Design review of the part built by this model. Coordinates are the model's own, in mm. A direction names the side the tool comes from. Round coordinates to 2 decimals unless told otherwise and drop trailing zeros. Order: outer loops, then holes, each group sorted by start corner. A loop starts at its lowest first (then second) coordinate and runs counter-clockwise, first axis right, second up. Notation, with made-up numbers: (83.25, -32) - (140.25, -32) arc R7 cw to (140.25, -22) - close; hole circle Ø6 at (62.5, 15). An arc over 180 degrees is marked (long way). Write item = value, one per line.
from build123d import *

# Parameters (mm, degrees)
SKETCH4_R           = 1.016
BOSS_EXTRUDE3_DEPTH = 8.382
BOSS_EXTRUDE4_DEPTH = 12.7
FILLET4_R           = 9.652


with BuildPart() as part:
    # Sketch4 → Boss-Extrude3 (new body)
    with BuildSketch(Plane(origin=(0, 0, 0), x_dir=(1, 0, 0), z_dir=(0, 1, 0))):
        with BuildLine():
            Line((-18.663003184, -7.371341), (-24.923761703, -4.89551862))
            ThreePointArc((-24.923761703, -4.89551862), (1.824176411, 25.334410994), (23.965300472, -8.415721794))
            Line((23.965300472, -8.415721794), (18.932587373, -6.648420217))
            ThreePointArc((18.932587373, -6.648420217), (7.011176439, 18.801270195), (-18.663003184, 7.371341))
            ThreePointArc((-18.663003184, 7.371341), (-7.821215551, 0), (-18.663003184, -7.371341))
        make_face()
        with Locations((-15.748, 0)):
            Circle(SKETCH4_R, mode=Mode.SUBTRACT)
    extrude(amount=BOSS_EXTRUDE3_DEPTH)

    # Sketch5 → Boss-Extrude4 (add)
    with BuildSketch(Plane.XZ):
        with BuildLine():
            Line((18.932587373, 6.648420217), (23.965300472, 8.415721794))
            ThreePointArc((23.965300472, 8.415721794), (24.582982591, -6.390380813), (16.83300832, -19.021299401))
            Line((16.83300832, -19.021299401), (13.298076573, -15.026826527))
            ThreePointArc((13.298076573, -15.026826527), (19.420556247, -5.048400842), (18.932587373, 6.648420217))
        make_face()
    extrude(amount=BOSS_EXTRUDE4_DEPTH)

    # Fillet4
    fillet4_edges = [part.edges().sort_by_distance(p)[0] for p in [
        (-24.923761703, 4.191, 4.89551862),
    ]]
    fillet(fillet4_edges, radius=FILLET4_R)


solid = part.part
1) The part is to be moulded in two halves that separate along X. For faces 1 (the flat face through (-13, 0, -6)), 2 (the cylindrical face through (-16.763, 4.132, -0.045)), 3 (the cylindrical face through (-23.97, 4.25, 3.07)), say which applies: released by +X, released by -X, zero draft, split by the parting line, or undercut.
Findings:
face_1 = zero draft
face_2 = undercut
face_3 = released by -X
2) We need section A-A on z = -16.5. Write out the cut boundary in (x, y), and give its area (3 significant figures).
Findings:
outline = (-19.31, 0) - (-11.42, 0) - (-11.42, 8.38) - (-19.31, 8.38) - close; (11.42, 0) - (14.6, 0) - (14.6, -12.7) - (19.31, -12.7) - (19.31, 8.38) - (11.42, 8.38) - close
area = 192 mm^2
3) To check wall thickness, follow L1, parallel to Z at x = -15, y = 7.25; L2, parallel to Z at x = -17, y = 6.25; L3, parallel to Y at x = 0, z = -23. State the ranges of each line that lie inside material, in increasing order. Write a range as from..to.
Findings:
L1 = -20.5..-13.33, -7.89..-0.69, 0.69..7.89
L2 = -18.87..-10.66, -7.83..7.83
L3 = 0..8.38
4) We need section C-C on z = 0. Write out the cut boundary in (x, y), and give its area (3 significant figures).
Findings:
outline = (-25.12, 0) - (-16.76, 0) - (-16.76, 8.38) - (-25.12, 8.38) - close; (-14.73, 0) - (-7.82, 0) - (-7.82, 8.38) - (-14.73, 8.38) - close; (20.07, -12.7) - (25.4, -12.7) - (25.4, 8.38) - (20.07, 8.38) - close
area = 240 mm^2
5) We need section D-D on x = 21. Write out the cut boundary in (y, z), and give its area (3 significant figures).
Findings:
outline = (-12.7, -14.29) - (8.38, -14.29) - (8.38, 7.37) - (-12.7, 7.37) - close
area = 457 mm^2
6) For faces 4 (the flat face through (21.41, -2.01, 7.52)), 5 (the flat face through (15.09, -6.26, -17.05)), 6 (the flat face through (21, -12.7, -5)), list the 3-axis set-ups (+Z, -Z, +X, -X, +Y, -Y) from which the entire face can be reached by the end or side of a thin tool; tool diameter is ignored.
Findings:
face_4 = +Z, +Y, -Y
face_5 = -Z, -X, -Y
face_6 = +Z, -Z, +X, -X, -Y
7) Clearance check with flat-ended pins moving along their axes: pin 1 Ø12 at (y, z) = (1.5, -18.5) entering from -X; pin 2 Ø1 at (y, z) = (2.5, -16.5) entering from +X; pin 3 Ø8 at (x, y) = (-16, -2) entering from +Z. State where each tip first meets the part, or that it passes through.
Findings:
pin_1 = -22.11
pin_2 = 19.73
pin_3 = 7.93
